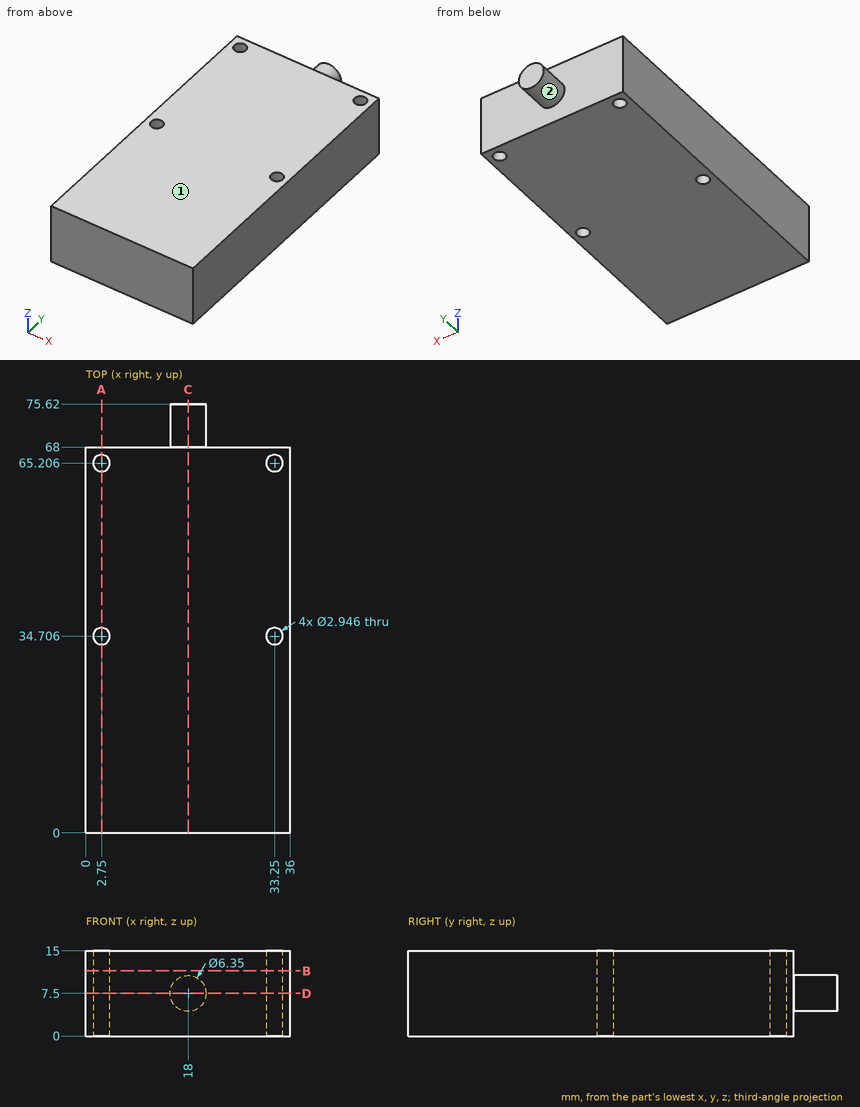
Verification items for this drawing (mm, ordinates from the low corner). A direction names the side the tool comes from. Round coordinates to 2 decimals unless told otherwise and drop trailing zeros. Write each loop counter-clockwise with the first axis right and the second up, starting at its lowest first coordinate (ties: lowest second). Pieces come first, ordered by that corner, then holes. Notation, with made-up numbers: M 85,72 L 127,72 A18 cw 127,98 Z; hole C 55.25,27.5 d10. An arc over 180 degrees is marked long. Write item = value, one per line. Start each with the question number.
1. Tool access check on the marked faces 1 and 2. Record the directions out of +Z, -Z, +X, -X, +Y, -Y that give a thin tool (end or side, any length) a straight path to the whole face; none if there is none.
2. Section check D-D, the plane z = 7.5. State how many separate pieces and enclosed holes the cut face has, then the cut area to 3 significant figures.
3. Gauge pin test, flat ends, axial feed: pin 1 (4.5 mm diameter, centred on x = 2.75, y = 65.206, fed in from -Z); pin 2 (1.8 mm diameter, centred on x = 2.75, y = 34.706, fed in from +Z); pin 3 (4.5 mm diameter, centred on x = 9.5, z = 8.5, fed in from +Y). Record the tip position at first contact, or that the pin passes through.
4. Scan lines: line 1 (Y direction, x = 33.25, z = 9.25); line 2 (X direction, y = 35, z = 11.5); line 3 (Y direction, x = 30.5, z = 8). Record each from-to range of solid material in increasing order. Write a range as [from, to].
5. Section check C-C, the plane x = 18. Record the cut outline in (y, z) (1 decimal).
6. Section check B-B, the plane z = 11.5. Record the cut outline in (x, y), then the cut area to 3 significant figures.
7. Section check A-A, the plane x = 2.75. Record the cut outline in (y, z).
Results found:
q1.face_1 = +Z, +X, -X, +Y, -Y
q1.face_2 = +Y
q2.separate_pieces = 1
q2.enclosed_holes = 4
q2.area = 2,470 mm^2
q3.pin_1 = 0
q3.pin_2 = through
q3.pin_3 = 68
q4.line_1 = [0, 33.23], [36.18, 63.73], [66.68, 68]
q4.line_2 = [0, 1.31], [4.19, 31.81], [34.69, 36]
q4.line_3 = [0, 68]
q5.outline = M 0,0 L 68,0 L 68,4.3 L 75.6,4.3 L 75.6,10.7 L 68,10.7 L 68,15 L 0,15 Z
q6.outline = M 0,0 L 36,0 L 36,68 L 0,68 Z; hole C 2.75,34.71 d2.95; hole C 2.75,65.21 d2.95; hole C 33.25,34.71 d2.95; hole C 33.25,65.21 d2.95
q6.area = 2,420 mm^2
q7.outline = M 0,0 L 33.23,0 L 33.23,15 L 0,15 Z; M 36.18,0 L 63.73,0 L 63.73,15 L 36.18,15 Z; M 66.68,0 L 68,0 L 68,15 L 66.68,15 Z
